For this review, take the finished solid that the model builds, in its own axes (mm). Round coordinates to 2 decimals unless told otherwise and drop trailing zeros. Write each loop counter-clockwise with the first axis right and the second up, starting at its lowest first coordinate (ties: lowest second). Pieces come first, ordered by that corner, then holes. Notation, with made-up numbers: M 42,22 L 57,22 A19 ccw 57,46 Z; hole C -12,62.5 d10. An arc over 180 degrees is marked long. Answer in a Markdown table with one row per item.
```python
from build123d import *

# Parameters (mm, degrees)
F0_R     = 2
F1_DEPTH = 3.2
F2_SIZE  = 3


with BuildPart() as f1:
    # F0 (on Top) → F1 (new body)
    with BuildSketch(Plane.XY):
        Polygon((-96, 131.9), (-123, 131.9), (-123, 117.5), (-127, 113.5), (-127, -112.732986), (-123, -117.5), (123, -117.5), (127, -112.732986), (127, 113.5), (123, 117.5), (-96, 117.5), align=None)
        with Locations((-104.5, -107.5)):
            Circle(F0_R, mode=Mode.SUBTRACT)
        with Locations((104.5, -107.5)):
            Circle(F0_R, mode=Mode.SUBTRACT)
        with Locations((0, -24)):
            Circle(F0_R, mode=Mode.SUBTRACT)
        with Locations((-104.5, 101.5)):
            Circle(F0_R, mode=Mode.SUBTRACT)
        with Locations((0, 17)):
            Circle(F0_R, mode=Mode.SUBTRACT)
        with Locations((104.5, 101.5)):
            Circle(F0_R, mode=Mode.SUBTRACT)
    extrude(amount=F1_DEPTH)

    # F2
    f2_edges = [f1.edges().sort_by_distance(p)[0] for p in [
        (-106.5, 101.5, 3.2),
        (-2, 17, 3.2),
        (-2, -24, 3.2),
        (102.5, 101.5, 3.2),
        (102.5, -107.5, 3.2),
        (-106.5, -107.5, 3.2),
    ]]
    chamfer(f2_edges, length=F2_SIZE)


solid = f1.part
```
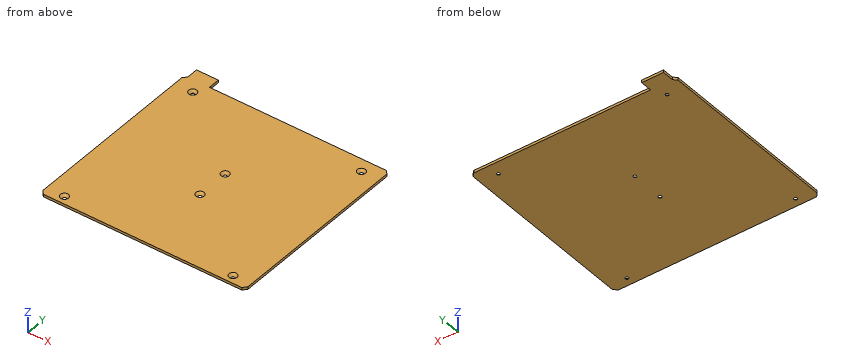
Q1. For probe 1 along Y at (x, z) = (0, 0.15); probe 2 along Y at (x, z) = (-104.5, 0.1); probe 3 along Y at (x, z) = (-44, 1.05), list the stretches that pass through material, from the lowest coordinate up.
Found:
| item | result |
|---|---|
| probe 1 | -117.5 to -26, -22 to 15, 19 to 117.5 |
| probe 2 | -117.5 to -109.5, -105.5 to 99.5, 103.5 to 131.9 |
| probe 3 | -117.5 to 117.5 |
Q2. Take a section at A-A (z = 1.2). State the section outline as (x, y) points, then the cut area to 3 significant figures.
Found:
| item | result |
|---|---|
| outline | M -127,-112.73 L -123,-117.5 L 123,-117.5 L 127,-112.73 L 127,113.5 L 123,117.5 L -96,117.5 L -96,131.9 L -123,131.9 L -123,117.5 L -127,113.5 Z; hole C -104.5,-107.5 d6; hole C -104.5,101.5 d6; hole C 0,-24 d6; hole C 0,17 d6; hole C 104.5,-107.5 d6; hole C 104.5,101.5 d6 |
| area | 59,900 mm² |
Q3. Insertion check: P1, Ø1.5, axis at x = 81, z = 1, coming from the +Y side; P2, Ø1, axis at y = 123, z = 2.5, coming from the -X side. Each pin has a flat end and moves straight along its axis. Give the tip position at first contact, or say it passes through.
Found:
| item | result |
|---|---|
| P1 | y = 117.5 |
| P2 | x = -123 |
Q4. Take a section at B-B (x = -68). State the section outline as (y, z) points.
Found:
| item | result |
|---|---|
| outline | M -117.5,0 L 117.5,0 L 117.5,3.2 L -117.5,3.2 Z |
